```python
from build123d import *

# Parameters (mm, degrees)
SKETCH1_W                                      = 45
SKETCH1_H                                      = 35
BOSS_EXTRUDE1_DEPTH                            = 3
CSK_FOR_M3_FLAT_HEAD_MACHINE_SCREW2_AT_2_COUNT = 2
CSK_FOR_M3_FLAT_HEAD_MACHINE_SCREW2_AT_2_PITCH = 20
CSK_FOR_M3_FLAT_HEAD_MACHINE_SCREW2_AT_3_COUNT = 2
CSK_FOR_M3_FLAT_HEAD_MACHINE_SCREW2_AT_3_PITCH = 28.284271247
CSK_FOR_M3_FLAT_HEAD_MACHINE_SCREW2_AT_4_COUNT = 2
CSK_FOR_M3_FLAT_HEAD_MACHINE_SCREW2_AT_4_PITCH = 20
SKETCH7_W                                      = 15
SKETCH7_H                                      = 4
BOSS_EXTRUDE2_DEPTH                            = 60
FILLET1_R                                      = 2


with BuildPart() as part:
    # Sketch1 → Boss-Extrude1 (new body)
    with BuildSketch(Plane(origin=(0, 0, 0), x_dir=(1, 0, 0), z_dir=(0, 1, 0))):
        Rectangle(SKETCH1_W, SKETCH1_H)
    extrude(amount=BOSS_EXTRUDE1_DEPTH)

    # Sketch5 → CSK for M3 Flat Head Machine Screw2 (revolve, cut)
    with BuildSketch(Plane(origin=(10, 3, -10), x_dir=(0, 0, 1), z_dir=(1, 0, 0))):
        Polygon((0, 0), (0, 3), (1.7, 3), (1.7, 1.45), (3.15, 0), align=None)
    csk_for_m3_flat_head_machine_screw2 = revolve(axis=Axis((10, 9.35, -10), (0, -1, 0)), mode=Mode.SUBTRACT)

    # CSK for M3 Flat Head Machine Screw2 at 2: CSK for M3 Flat Head Machine Screw2 ×2
    with Locations(*[(-i * CSK_FOR_M3_FLAT_HEAD_MACHINE_SCREW2_AT_2_PITCH, 0, 0) for i in range(1, CSK_FOR_M3_FLAT_HEAD_MACHINE_SCREW2_AT_2_COUNT)]):
        add(csk_for_m3_flat_head_machine_screw2, mode=Mode.SUBTRACT)

    # CSK for M3 Flat Head Machine Screw2 at 3: CSK for M3 Flat Head Machine Screw2 ×2
    with Locations(*[Vector(-0.707106781, 0, 0.707106781) * (i * CSK_FOR_M3_FLAT_HEAD_MACHINE_SCREW2_AT_3_PITCH) for i in range(1, CSK_FOR_M3_FLAT_HEAD_MACHINE_SCREW2_AT_3_COUNT)]):
        add(csk_for_m3_flat_head_machine_screw2, mode=Mode.SUBTRACT)

    # CSK for M3 Flat Head Machine Screw2 at 4: CSK for M3 Flat Head Machine Screw2 ×2
    with Locations(*[(0, 0, i * CSK_FOR_M3_FLAT_HEAD_MACHINE_SCREW2_AT_4_PITCH) for i in range(1, CSK_FOR_M3_FLAT_HEAD_MACHINE_SCREW2_AT_4_COUNT)]):
        add(csk_for_m3_flat_head_machine_screw2, mode=Mode.SUBTRACT)

    # Sketch7 → Boss-Extrude2 (add, along a direction that is not the sketch's normal)
    with BuildSketch(Plane(origin=(0, 3, 0), x_dir=(1, 0, 0), z_dir=(0, 1, 0))):
        Rectangle(SKETCH7_W, SKETCH7_H)
    extrude(amount=BOSS_EXTRUDE2_DEPTH, dir=(0, 0.866025404, -0.5))

    # Fillet1
    fillet1_edges = [part.edges().sort_by_distance(p)[0] for p in [
        (22.5, 3, 0),
        (0, 3, -17.5),
        (-22.5, 3, 0),
        (0, 3, 17.5),
        (-22.5, 1.5, -17.5),
        (22.5, 1.5, -17.5),
        (22.5, 1.5, 17.5),
        (-22.5, 1.5, 17.5),
    ]]
    fillet(fillet1_edges, radius=FILLET1_R)


solid = part.part
```
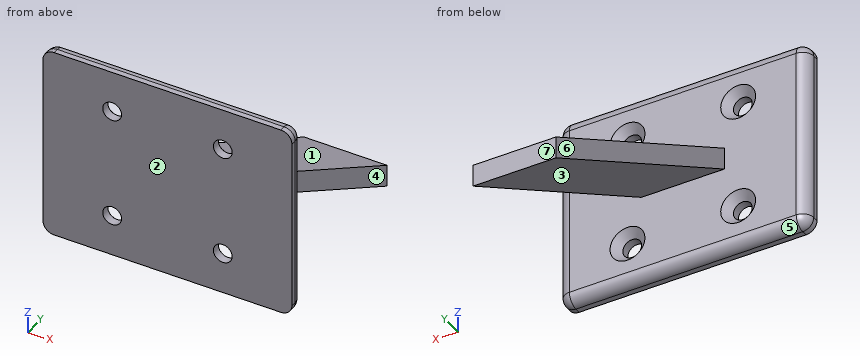
Design review of the part built by this model. Coordinates are the model's own, in mm. Face numbers are marked on the shaded views. A direction names the side the tool comes from. Give positions to 0.01 mm unless a question says otherwise; leave off trailing zeros. Order: outer loops, then holes, each group sorted by start corner. A loop starts at its lowest first (then second) coordinate and runs counter-clockwise, first axis right, second up. Notation, with made-up numbers: M 4.5,79.5 L 39.5,79.5 A14 ccw 39.5,103.5 Z; hole C 21,53.5 d6. An arc over 180 degrees is marked long. One line per question, with ' | ' between items. Start each with the question number.
Q1. The part is to be moulded in two halves that separate along Y. For the marked faces 1, 2, 3 and 4, say which applies: +Y half, -Y half, draft (parallel to the pull), parting line (faces both ways), or undercut.
Q2. We need section A-A (x = 10). Write out the cut boundary in (y, z).
Q3. We need section B-B (z = 10). Write out the cut boundary in (x, y).
Q4. Machinability: for the marked faces 5, 6 and 7, which of the approach directions +Z, -Z, +X, -X, +Y, -Y give a long, thin tool a straight path to every point of the face, cutting with its end or side? Answer none if there is none.
Q5. We need section D-D (z = -5). Write out the cut boundary in (x, y).
Q6. For L1, parallel to X at y = 0.9, z = -10; L2, parallel to Z at x = 10, y = 0.75; L3, parallel to Y at x = 11, z = -7, list the stretches that pass through material, from the lowest coordinate up. Write a range as [from, to].
Q7. For pin 1 Ø10 at (x, y) = (-15, 24) entering from -Z; pin 2 Ø4 at (x, y) = (-1, 48) entering from -Z; pin 3 Ø1 at (x, z) = (3.5, 7) entering from +Y; pin 4 Ø6 at (y, z) = (16.5, -9.5) entering from -X, all flat-tipped, find the tip position at first contact; note any pin that passes through.
Q8. We need section C-C (x = -2.5). Write out the cut boundary in (y, z).
Returned:
1) face 1: +Y half | face 2: -Y half | face 3: undercut | face 4: draft
2) outline: M 0,-17.5 L 1,-17.5 A2 ccw 3,-15.5 L 3,-13.15 L 1.55,-11.7 L 0,-11.7 Z; M 0,-8.3 L 1.55,-8.3 L 3,-6.85 L 3,6.85 L 1.55,8.3 L 0,8.3 Z; M 0,11.7 L 1.55,11.7 L 3,13.15 L 3,15.5 A2 ccw 1,17.5 L 0,17.5 Z
3) outline: M -22.5,0 L -11.7,0 L -11.7,1.55 L -13.15,3 L -20.5,3 A2 ccw -22.5,1 Z; M -8.3,0 L 8.3,0 L 8.3,1.55 L 6.85,3 L -6.85,3 L -8.3,1.55 Z; M 11.7,0 L 22.5,0 L 22.5,1 A2 ccw 20.5,3 L 13.15,3 L 11.7,1.55 Z
4) face 5: -Z, +X, -X | face 6: +Z, -Z, -X, +Y | face 7: +Z, -Z, +X, -X, +Y
5) outline: M -22.5,0 L 22.5,0 L 22.5,1 A2 ccw 20.5,3 L -20.5,3 A2 ccw -22.5,1 Z; M -7.5,8.2 L 7.5,8.2 L 7.5,15.12 L -7.5,15.12 Z
6) L1: [-22.5, -11.7], [-8.3, 8.3], [11.7, 22.5] | L2: [-17.5, -11.7], [-8.3, 8.3], [11.7, 17.5] | L3: [0, 3]
7) pin 1: through | pin 2: z = -29.14 | pin 3: y = 3 | pin 4: x = -7.5
8) outline: M 0,-17.5 L 1,-17.5 A2 ccw 3,-15.5 L 3,-2 L 54.96,-32 L 54.96,-28 L 3,2 L 3,15.5 A2 ccw 1,17.5 L 0,17.5 Z
